```python
from build123d import *

# Parameters (mm, degrees)
F0_R     = 100.33
F0_R_2   = 43.815
F1_DEPTH = 6.35
F1_TAPER = -3
F2_DEPTH = 2.54
F3_R     = 43.4822106016
F4_DEPTH = 3.81
F3_R_2   = 99.3927893984
F3_R_3   = 45.085
F5_DEPTH = 3.81
F5_TAPER = 8


with BuildPart() as f1:
    # F0 (on Top) → F1 (new body)
    with BuildSketch(Plane.XY):
        Circle(F0_R)
        Circle(F0_R_2, mode=Mode.SUBTRACT)
    extrude(amount=F1_DEPTH, taper=F1_TAPER)

    # F0 (on Top) → F2 (join)
    with BuildSketch(Plane.XY):
        Circle(F0_R_2)
    extrude(amount=F2_DEPTH)

    # F3 (on face) → F4 (cut, through all)
    with BuildSketch(Plane.XY.offset(6.35)):
        Circle(F3_R)
    extrude(amount=-F4_DEPTH, mode=Mode.SUBTRACT)

    # F3 (on face) → F5 (cut, through all)
    with BuildSketch(Plane.XY.offset(6.35)):
        Circle(F3_R_2)
        Circle(F3_R_3, mode=Mode.SUBTRACT)
    extrude(amount=-F5_DEPTH, taper=F5_TAPER, mode=Mode.SUBTRACT)


solid = f1.part
```
For this review, take the finished solid that the model builds, in its own axes (mm). A direction names the side the tool comes from. Give positions to 0.01 mm unless a question says otherwise; leave off trailing zeros. Write each loop counter-clockwise with the first axis right and the second up, starting at its lowest first coordinate (ties: lowest second). Pieces come first, ordered by that corner, then holes.
Item 1: Take a section at B-B (x = 0). Give the boundary of the cut face in (y, z) (3 decimals).
Item 2: The part is to be moulded in two halves that separate along X. For faces 3 (the face through (95.717, 30.143, 0.397)), 4 (the face through (43, -21, 2.54)), 5 (the face through (-1, 1, 0)), say which applies: +X half, -X half, draft (parallel to the pull), parting line (faces both ways), or undercut.
Item 3: Wall thickness on probe 1 along X at (y, z) = (-29, 3.25); probe 2 along X at (y, z) = (-17.5, 3.25); probe 3 along Y at (x, z) = (-34.5, 3): over which ranges is each line inside the solid? List them lowest first.
Item 4: Take a section at A-A (z = 3.75). Give the boundary of the cut face in (x, y).
Item 5: Insertion check: P1, Ø1.5, axis at x = 76, y = 6.5, coming from the +Z side; P2, Ø1.5, axis at x = -39, z = 5.5, coming from the -Y side. Each pin has a flat end and moves straight along its axis. Give the tip position at first contact, or say it passes through.
Item 6: Machinability: for faces 1 (the face through (-9.781, 44.046, 6.112)), 2 (the face through (41.484, -13.064, 6.165)), which of the approach directions +Z, -Z, +X, -X, +Y, -Y give a long, thin tool a straight path to every point of the face, cutting with its end or side? Answer none if there is none.
Established:
1. outline: (-100.663, 6.35) - (-100.33, 0) - (100.33, 0) - (100.663, 6.35) - (99.393, 6.35) - (98.857, 2.54) - (45.62, 2.54) - (45.085, 6.35) - (43.482, 6.35) - (43.682, 2.54) - (-43.682, 2.54) - (-43.482, 6.35) - (-45.085, 6.35) - (-45.62, 2.54) - (-98.857, 2.54) - (-99.393, 6.35) - close
2. face 3: parting line
2. face 4: undercut
2. face 5: draft
3. probe 1: x = -96.23 to -94.61, -35.09 to -32.62, 32.62 to 35.09, 94.61 to 96.23
3. probe 2: x = -98.96 to -97.4, -42.02 to -39.98, 39.98 to 42.02, 97.4 to 98.96
3. probe 3: y = -94.38 to -92.71, -29.75 to -26.75, 26.75 to 29.75, 92.71 to 94.38
4. outline: circle Ø201.05 at (0, 0); circle Ø90.9 at (0, 0); hole circle Ø198.05 at (0, 0); hole circle Ø87.24 at (0, 0)
5. P1: stops at z = 2.54
5. P2: stops at y = -93.07
6. face 1: +Z
6. face 2: none
